The listing builds one solid part. Answer for the finished solid, in the listing's coordinates (mm). Face numbers are marked on the shaded views. A direction names the side the tool comes from. Coordinates: 2 decimals unless noted, no trailing zeros. Order: outer loops, then holes, each group sorted by start corner. A loop starts at its lowest first (then second) coordinate and runs counter-clockwise, first axis right, second up. Notation, with made-up numbers: (40.5, 39) -> (75.5, 39) arc R20 ccw to (75.5, 74) -> close; hole circle Ø11 at (25.25, -8.5). An arc over 180 degrees is marked (long way). Answer in a Markdown table with one row per item. Add a question column.
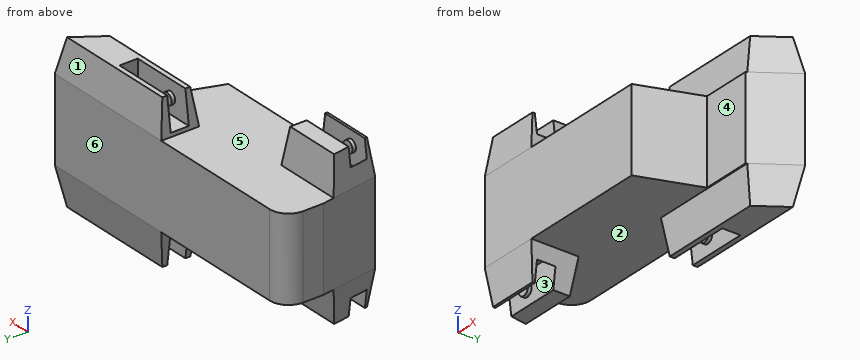
```python
from build123d import *

# Parameters (mm, degrees)
SALIENTE_EXTRUIR1_DEPTH           = 35
SALIENTE_EXTRUIR2_DEPTH           = 15
SALIENTE_EXTRUIR2_DRAFT           = 8
SALIENTE_EXTRUIR2_PROFILE_2_DEPTH = 15
SALIENTE_EXTRUIR2_PROFILE_2_DRAFT = 8
SIMETR_A1_COPY_1_DEPTH            = 15
SIMETR_A1_COPY_1_DRAFT            = 8
SIMETR_A1_COPY_2_DEPTH            = 15
SIMETR_A1_COPY_2_DRAFT            = 8
SIMETR_A1_COPY_3_DEPTH            = 15
SIMETR_A1_COPY_3_DRAFT            = 8
CROQUIS6_W                        = 28.054373897
CROQUIS6_H                        = 7.683774959
CORTAR_EXTRUIR2_DEPTH             = 13.5
CROQUIS8_R                        = 2.45
SALIENTE_EXTRUIR3_DEPTH           = 1.5
CROQUIS9_R                        = 2.45
SALIENTE_EXTRUIR4_DEPTH           = 1.5
CROQUIS10_R                       = 2.45
SALIENTE_EXTRUIR5_DEPTH           = 1.5
SALIENTE_EXTRUIR6_START           = 1.5
CROQUIS13_R                       = 2.45
SALIENTE_EXTRUIR6_DEPTH           = 1.5


with BuildPart() as part:
    # Croquis2 → Saliente-Extruir1 (new body)
    with BuildSketch(Plane.XY):
        with BuildLine():
            Line((30.877885102, -17.110048254), (39.667083018, 7.889951746))
            Line((39.667083018, 7.889951746), (60.667083018, 7.889951746))
            Line((60.667083018, 7.889951746), (71.969737573, 24.389951746))
            Line((71.969737573, 24.389951746), (-45.030262427, 24.389951746))
            ThreePointArc((-45.030262427, 24.389951746), (-50.687116676, 22.046805996), (-53.030262427, 16.389951746))
            Line((-53.030262427, 16.389951746), (-53.030262427, 7.889951746))
            Line((-53.030262427, 7.889951746), (-49.122114898, -17.110048254))
            Line((-49.122114898, -17.110048254), (30.877885102, -17.110048254))
        make_face()
    extrude(amount=SALIENTE_EXTRUIR1_DEPTH)


with BuildPart() as saliente_extruir2_tool:
    # Croquis5 → Saliente-Extruir2 (with draft: the straight prism first)
    with BuildSketch(Plane.XY.offset(35)):
        Polygon((-49.122114898, -17.110048254), (-23.748632921, -17.110048254), (-23.748632921, 2.889951746), (-52.248632921, 2.889951746), align=None)
    extrude(amount=SALIENTE_EXTRUIR2_DEPTH)
    # Saliente-Extruir2: the draft: its side faces are tilted about the plane it starts from
    saliente_extruir2_sides = [saliente_extruir2_tool.faces().sort_by_distance(p)[0] for p in [
        (-36.435373909, -17.110048254, 42.5),
        (-23.748632921, -7.110048254, 42.5),
        (-37.998632921, 2.889951746, 42.5),
        (-50.685373909, -7.110048254, 42.5),
    ]]
    draft(saliente_extruir2_sides, Plane.XY.offset(35), SALIENTE_EXTRUIR2_DRAFT)


with BuildPart() as part_1:
    add(part.part)

    # Saliente-Extruir2: add saliente_extruir2_tool
    add(saliente_extruir2_tool.part)


with BuildPart() as saliente_extruir2_profile_2_tool:
    # Croquis5 → Saliente-Extruir2 profile 2 (with draft: the straight prism first)
    with BuildSketch(Plane.XY.offset(35)):
        Polygon((71.969737573, 24.389951746), (13.969737573, 24.389951746), (13.969737573, 8.389951746), (61.009587702, 8.389951746), align=None)
    extrude(amount=SALIENTE_EXTRUIR2_PROFILE_2_DEPTH)
    # Saliente-Extruir2 profile 2: the draft: its side faces are tilted about the plane it starts from
    saliente_extruir2_profile_2_sides = [saliente_extruir2_profile_2_tool.faces().sort_by_distance(p)[0] for p in [
        (42.969737573, 24.389951746, 42.5),
        (13.969737573, 16.389951746, 42.5),
        (37.489662638, 8.389951746, 42.5),
        (66.489662638, 16.389951746, 42.5),
    ]]
    draft(saliente_extruir2_profile_2_sides, Plane.XY.offset(35), SALIENTE_EXTRUIR2_PROFILE_2_DRAFT)


with BuildPart() as part_2:
    add(part_1.part)

    # Saliente-Extruir2 profile 2: add saliente_extruir2_profile_2_tool
    add(saliente_extruir2_profile_2_tool.part)


with BuildPart() as simetr_a1_copy_1_tool:
    # Simetría1 copy 1 sketch → Simetría1 copy 1 (with draft: the straight prism first)
    with BuildSketch(Plane(origin=(0, 0, 0), x_dir=(1, 0, 0), z_dir=(0, 0, -1))):
        Polygon((-49.122114898, 17.110048254), (-23.748632921, 17.110048254), (-23.748632921, -2.889951746), (-52.248632921, -2.889951746), align=None)
    extrude(amount=SIMETR_A1_COPY_1_DEPTH)
    # Simetría1 copy 1: the draft: its side faces are tilted about the plane it starts from
    simetr_a1_copy_1_sides = [simetr_a1_copy_1_tool.faces().sort_by_distance(p)[0] for p in [
        (-36.435373909, -17.110048254, -7.5),
        (-23.748632921, -7.110048254, -7.5),
        (-37.998632921, 2.889951746, -7.5),
        (-50.685373909, -7.110048254, -7.5),
    ]]
    draft(simetr_a1_copy_1_sides, Plane(origin=(0, 0, 0), x_dir=(1, 0, 0), z_dir=(0, 0, -1)), SIMETR_A1_COPY_1_DRAFT)


with BuildPart() as part_3:
    add(part_2.part)

    # Simetría1 copy 1: add simetr_a1_copy_1_tool
    add(simetr_a1_copy_1_tool.part)


with BuildPart() as simetr_a1_copy_2_tool:
    # Simetría1 copy 2 sketch → Simetría1 copy 2 (with draft: the straight prism first)
    with BuildSketch(Plane(origin=(0, 0, 0), x_dir=(1, 0, 0), z_dir=(0, 0, -1))):
        Polygon((71.969737573, -24.389951746), (13.969737573, -24.389951746), (13.969737573, -8.389951746), (61.009587702, -8.389951746), align=None)
    extrude(amount=SIMETR_A1_COPY_2_DEPTH)
    # Simetría1 copy 2: the draft: its side faces are tilted about the plane it starts from
    simetr_a1_copy_2_sides = [simetr_a1_copy_2_tool.faces().sort_by_distance(p)[0] for p in [
        (42.969737573, 24.389951746, -7.5),
        (13.969737573, 16.389951746, -7.5),
        (37.489662638, 8.389951746, -7.5),
        (66.489662638, 16.389951746, -7.5),
    ]]
    draft(simetr_a1_copy_2_sides, Plane(origin=(0, 0, 0), x_dir=(1, 0, 0), z_dir=(0, 0, -1)), SIMETR_A1_COPY_2_DRAFT)


with BuildPart() as part_4:
    add(part_3.part)

    # Simetría1 copy 2: add simetr_a1_copy_2_tool
    add(simetr_a1_copy_2_tool.part)


with BuildPart() as simetr_a1_copy_3_tool:
    # Simetría1 copy 3 sketch → Simetría1 copy 3 (with draft: the straight prism first)
    with BuildSketch(Plane(origin=(0, 0, 0), x_dir=(1, 0, 0), z_dir=(0, 0, -1))):
        Polygon((71.969737573, -24.389951746), (13.969737573, -24.389951746), (13.969737573, -8.389951746), (61.009587702, -8.389951746), align=None)
    extrude(amount=SIMETR_A1_COPY_3_DEPTH)
    # Simetría1 copy 3: the draft: its side faces are tilted about the plane it starts from
    simetr_a1_copy_3_sides = [simetr_a1_copy_3_tool.faces().sort_by_distance(p)[0] for p in [
        (42.969737573, 24.389951746, -7.5),
        (13.969737573, 16.389951746, -7.5),
        (37.489662638, 8.389951746, -7.5),
        (66.489662638, 16.389951746, -7.5),
    ]]
    draft(simetr_a1_copy_3_sides, Plane(origin=(0, 0, 0), x_dir=(1, 0, 0), z_dir=(0, 0, -1)), SIMETR_A1_COPY_3_DRAFT)


with BuildPart() as part_5:
    add(part_4.part)

    # Simetría1 copy 3: add simetr_a1_copy_3_tool
    add(simetr_a1_copy_3_tool.part)

    # Croquis6 → Cortar-Extruir2 (cut)
    with BuildSketch(Plane(origin=(0, 0, -15), x_dir=(-1, 0, 0), z_dir=(0, 0, -1))):
        with Locations((-27.996924522, 16.389951747)):
            Rectangle(CROQUIS6_W, CROQUIS6_H)
        Polygon((24.660477495, -6.201935733), (49.760477495, -6.201935733), (48.541135466, -14.001935733), (24.660477495, -14.001935733), align=None)
    cortar_extruir2 = extrude(amount=-CORTAR_EXTRUIR2_DEPTH, mode=Mode.SUBTRACT)

    # Simetría2: Cortar-Extruir2 across plane
    add(cortar_extruir2.mirror(Plane(origin=(0, 0, 17.5), x_dir=(1, 0, 0), z_dir=(0, 0, -1))), mode=Mode.SUBTRACT)

    # Croquis8 → Saliente-Extruir3 (add)
    with BuildSketch(Plane.XZ.offset(-20.231839226)):
        with Locations((24.182512404, 43)):
            Circle(CROQUIS8_R)
    saliente_extruir3 = extrude(amount=SALIENTE_EXTRUIR3_DEPTH)

    # Simetría3: Saliente-Extruir3 across plane
    add(saliente_extruir3.mirror(Plane(origin=(0, 0, 17.5), x_dir=(1, 0, 0), z_dir=(0, 0, -1))))

    # Croquis9 → Saliente-Extruir4 (add)
    with BuildSketch(Plane(origin=(0, 12.548064267, 0), x_dir=(1, 0, 0), z_dir=(0, 1, 0))):
        with Locations(Location((24.125726568, -43, 0), (0, 0, 180))):
            Circle(CROQUIS9_R)
    saliente_extruir4 = extrude(amount=SALIENTE_EXTRUIR4_DEPTH)

    # Simetría4: Saliente-Extruir4 across plane
    add(saliente_extruir4.mirror(Plane(origin=(0, 0, 17.5), x_dir=(1, 0, 0), z_dir=(0, 0, -1))))

    # Croquis10 → Saliente-Extruir5 (add)
    with BuildSketch(Plane.XZ.offset(6.201935733)):
        with Locations(Location((-40.160914021, 44, 0), (0, 0, 270))):
            Circle(CROQUIS10_R)
    saliente_extruir5 = extrude(amount=SALIENTE_EXTRUIR5_DEPTH)

    # Simetría5: Saliente-Extruir5 across plane
    add(saliente_extruir5.mirror(Plane(origin=(0, 0, 17.5), x_dir=(1, 0, 0), z_dir=(0, 0, -1))))

    # Croquis13 → Saliente-Extruir6 (add)
    with BuildSketch(Plane(origin=(0, -14.001935733, 0), x_dir=(1, 0, 0), z_dir=(0, 1, 0)).offset(SALIENTE_EXTRUIR6_START)):
        with Locations(Location((-40.160914021, -44, 0), (0, 0, 90))):
            Circle(CROQUIS13_R)
    saliente_extruir6 = extrude(amount=-SALIENTE_EXTRUIR6_DEPTH)

    # Simetría6: Saliente-Extruir6 across plane
    add(saliente_extruir6.mirror(Plane(origin=(0, 0, 17.5), x_dir=(1, 0, 0), z_dir=(0, 0, -1))))


solid = part_5.part
```
Q1. A cutting plane is placed at B-B (x = -18.5). Determine the outline of the cut face in (y, z).
Q2. For the marked faces 4, 5 and 6, determine the directions among +Z, -Z, +X, -X, +Y, -Y from which every point of the face is accessible in a straight line to the end or side of a thin tool.
Q3. A cutting plane is placed at A-A (z = 22). Determine the outline of the cut face in (x, y), then the cut area to 3 significant figures.
Q4. Given pin 1 (11 mm diameter, centred on x = -32, z = -8.5, fed in from -Y); pin 2 (6 mm diameter, centred on y = -6.5, z = 6, fed in from -X); pin 3 (6.5 mm diameter, centred on x = 55, z = 22, fed in from -Y); pin 4 (8 mm diameter, centred on y = 6.5, z = 16, fed in from -X), each flat-ended and moving along its own axis, determine where each tip first touches the part or whether it passes through.
Q5. A cutting plane is placed at C-C (y = 6.5). Determine the outline of the cut face in (x, z).
Q6. Determine the mould class of the marked faces 1, 2 and 3 for opening direction Y: +Y half, -Y half, draft (parallel to the pull), parting line (faces both ways), or undercut.
Q7. Straight lines are drawn through the part: line 1 (Z direction, x = 31, y = -11); line 2 (Y direction, x = 58, z = 22); line 3 (Z direction, x = -46.5, y = -7). For each, find the intervals that lie inside material, in ascending order.
Returned:
| question | item | result |
|---|---|---|
| 1 | outline | (-17.11, 0) -> (24.39, 0) -> (24.39, 35) -> (-17.11, 35) -> close |
| 2 | face 4 | +Z, -Z, +X, -Y |
| 2 | face 5 | +Z |
| 2 | face 6 | +Z, -Z, +X, -X, +Y |
| 3 | outline | (-53.03, 7.89) -> (-49.12, -17.11) -> (30.88, -17.11) -> (39.67, 7.89) -> (60.67, 7.89) -> (71.97, 24.39) -> (-45.03, 24.39) arc R8 ccw to (-53.03, 16.39) -> close |
| 3 | area | 4,110 mm² |
| 4 | pin 1 | stops at y = -16.69 |
| 4 | pin 2 | stops at x = -51.25 |
| 4 | pin 3 | stops at y = 7.89 |
| 4 | pin 4 | stops at x = -53.03 |
| 5 | outline | (-52.81, 0) -> (39.18, 0) -> (39.18, 35) -> (-52.81, 35) -> close |
| 6 | face 1 | +Y half |
| 6 | face 2 | draft |
| 6 | face 3 | undercut |
| 7 | line 1 | z = 0 to 35 |
| 7 | line 2 | y = 7.89 to 24.39 |
| 7 | line 3 | z = -1.5 to 36.5 |
